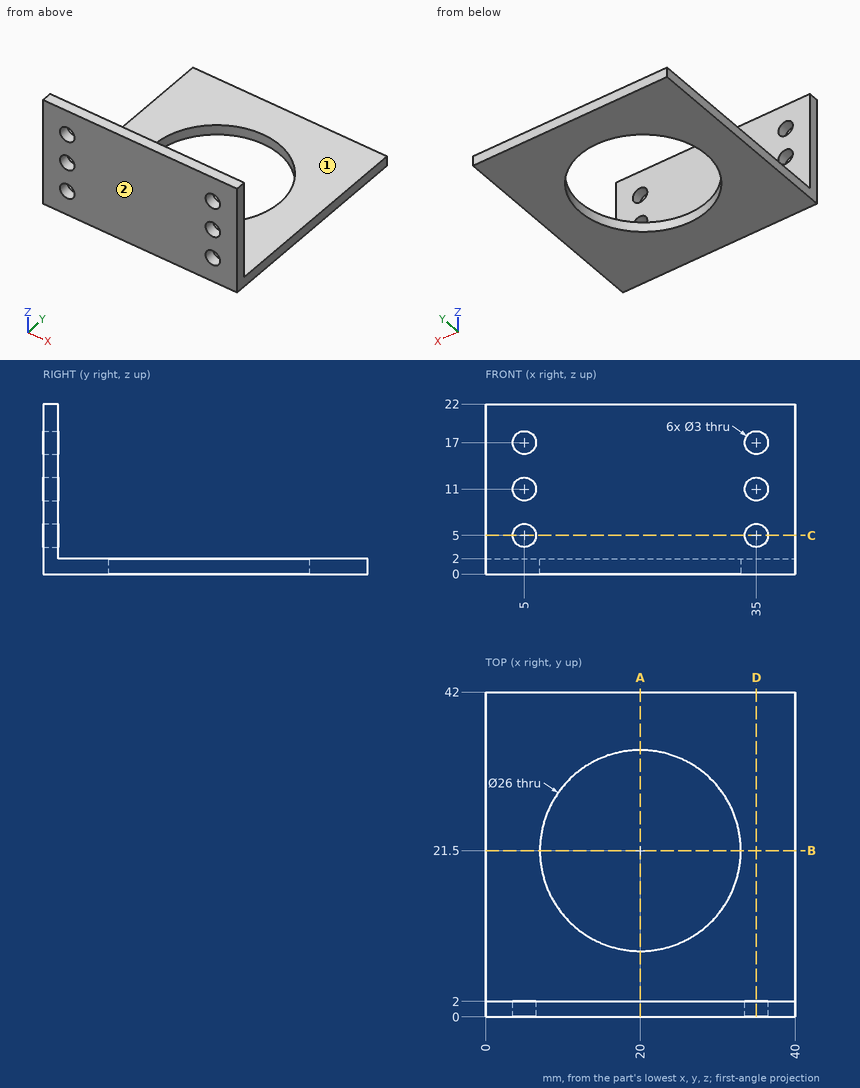
Study the drawing (mm; zero at the part's minimum x, y, z) and answer. A direction names the side the tool comes from. Give positions to 0.01 mm unless a question says otherwise; leave off trailing zeros. Loops run counter-clockwise (first coordinate to the right, second up) from the corner with the lowest first, then second, coordinate; pieces in that order, holes last. Notation, with made-up numbers: M 16,-8.75 L 59,-8.75 A7 ccw 59,2.25 Z; hole C 85.5,13.5 d2. An arc over 180 degrees is marked long. Answer as CSV lines item,"result".
Item 1: Given pin 1 Ø2.5 at (x, z) = (5, 5) entering from +Y; pin 2 Ø4 at (x, z) = (5, 17) entering from +Y; pin 3 Ø12 at (x, z) = (7, 5.5) entering from +Y, each flat-ended and moving along its own axis, determine where each tip first touches the part or whether it passes through.
Values follow:
pin 1,"passes through"
pin 2,"stops at y = 2"
pin 3,"stops at y = 42"
Item 2: The part is cut by section B-B (y = 21.5). Give the vertices of the cut face in (x, z), and give its area (3 significant figures).
Values follow:
outline,"M 0,0 L 7,0 L 7,2 L 0,2 Z; M 33,0 L 40,0 L 40,2 L 33,2 Z"
area,"28.0 mm^2"
Item 3: Straight lines are drawn through the part: line 1 along Z through (x, y) = (5, 1); line 2 along X through (y, z) = (1, 5); line 3 along Y through (x, z) = (20, 0.8). For each, find the intervals that lie inside material, in ascending order. Write a range as [from, to].
Values follow:
line 1,"z = [0, 3.5], [6.5, 9.5], [12.5, 15.5], [18.5, 22]"
line 2,"x = [0, 3.5], [6.5, 33.5], [36.5, 40]"
line 3,"y = [0, 8.5], [34.5, 42]"
Item 4: The part is cut by section C-C (z = 5). Give the vertices of the cut face in (x, y), and give its area (3 significant figures).
Values follow:
outline,"M 0,0 L 3.5,0 L 3.5,2 L 0,2 Z; M 6.5,0 L 33.5,0 L 33.5,2 L 6.5,2 Z; M 36.5,0 L 40,0 L 40,2 L 36.5,2 Z"
area,"68.0 mm^2"
Item 5: Which of the six approach directions +Z, -Z, +X, -X, +Y, -Y give full straight-line access (tool end or side, diameter ignored) to the marked faces 1 and 2?
Values follow:
face 1,"+Z, +X, -X, +Y"
face 2,"+Z, -Z, +X, -X, -Y"
Item 6: The part is cut by section A-A (x = 20). Give the vertices of the cut face in (y, z), and give its area (3 significant figures).
Values follow:
outline,"M 0,0 L 8.5,0 L 8.5,2 L 2,2 L 2,22 L 0,22 Z; M 34.5,0 L 42,0 L 42,2 L 34.5,2 Z"
area,"72.0 mm^2"
Item 7: The part is cut by section D-D (x = 35). Give the vertices of the cut face in (y, z), and give its area (3 significant figures).
Values follow:
outline,"M 0,0 L 42,0 L 42,2 L 2,2 L 2,3.5 L 0,3.5 Z; M 0,6.5 L 2,6.5 L 2,9.5 L 0,9.5 Z; M 0,12.5 L 2,12.5 L 2,15.5 L 0,15.5 Z; M 0,18.5 L 2,18.5 L 2,22 L 0,22 Z"
area,"106 mm^2"
